Source: CAD feature listing. Evaluate the final solid. Frame: model axes, mm. Coordinates: 2 decimals unless noted, no trailing zeros. Loops run counter-clockwise (first coordinate to the right, second up) from the corner with the lowest first, then second, coordinate; pieces in that order, holes last. Notation, with made-up numbers: (69.25, 59.5) -> (117.25, 59.5) arc R23 ccw to (117.25, 79.5) -> close; hole circle Ø4 at (13.5, 29). An arc over 180 degrees is marked (long way). One line per question, with ' | ' between items. Start each with the question number.
```python
from build123d import *

# Parameters (mm, degrees)
SKETCH1_R           = 38.1
SKETCH1_R_2         = 36.83
BOSS_EXTRUDE1_DEPTH = 254
CUT_EXTRUDE1_DEPTH  = 260.652113413
CIRPATTERN1_COUNT   = 2
CIRPATTERN1_ANGLE   = 90


with BuildPart() as part:
    # Sketch1 → Boss-Extrude1 (new body)
    with BuildSketch(Plane(origin=(0, 0, 0), x_dir=(1, 0, 0), z_dir=(0, 1, 0))):
        with Locations(Location((0, 0, 0), (0, 0, 270))):
            Circle(SKETCH1_R)
        with Locations(Location((0, 0, 0), (0, 0, 270))):
            Circle(SKETCH1_R_2, mode=Mode.SUBTRACT)
    extrude(amount=BOSS_EXTRUDE1_DEPTH)

    # Sketch2 → Cut-Extrude1 (cut, symmetric)
    with BuildSketch(Plane.XY):
        with BuildLine():
            Line((-1.61925, 12.7), (-1.61925, 107.823))
            ThreePointArc((-1.61925, 107.823), (0, 109.44225), (1.61925, 107.823))
            Line((1.61925, 107.823), (1.61925, 12.7))
            ThreePointArc((1.61925, 12.7), (0, 11.08075), (-1.61925, 12.7))
        make_face()
    cut_extrude1 = extrude(amount=CUT_EXTRUDE1_DEPTH, both=True, mode=Mode.SUBTRACT)

    # CirPattern1: Cut-Extrude1 ×2 about axis
    cirpattern1_axis = Axis((0, -12.7, 0), (0, 1, 0))
    for i in range(1, CIRPATTERN1_COUNT):
        add(cut_extrude1.rotate(cirpattern1_axis, i * CIRPATTERN1_ANGLE / (CIRPATTERN1_COUNT - 1)), mode=Mode.SUBTRACT)


solid = part.part
```
(1) Draft query along Z for faces 1 (the cylindrical face through (-23.183, 125.222, -30.235)), 2 (the cylindrical face through (-22.41, 125.222, -29.227)), 3 (the flat face through (31.2, 0, -19.9)). Return one class per face: pulls with the +Z half, pulls with the -Z half, needs draft (parallel to the pull), parting line crosses it, or undercut.
(2) Cut plane A-A, the plane y = 95. Return the cut outline in (x, z).
(3) Cut plane B-B, the plane x = 16. Return the cut outline in (y, z).
(4) Contact query for flat-ended pins moving along their axis: pin 1 Ø1.5 at (y, z) = (83.5, 24) entering from -X; pin 2 Ø12 at (x, y) = (-17.5, 81) entering from +Z; pin 3 Ø12 at (y, z) = (227.5, 27.5) entering from +X. Output: stop coordinate, or through.
(5) Cut plane C-C, the plane z = 33. Return the cut outline in (x, y), and give its area (3 significant figures).
(6) Ray query, L1, parallel to X at y = 141, z = 0; L2, parallel to X at y = 66.5, z = 24. Return the intervals inside material, ascending.
(7) Cut plane D-D, the plane y = 208.5. Return the cut outline in (x, z).
Here are the results:
1) face 1: parting line crosses it | face 2: undercut | face 3: needs draft
2) outline: (-38.07, -1.62) arc R38.1 ccw to (-1.62, -38.07) -> (-1.62, -36.79) arc R36.83 cw to (-36.79, -1.62) -> close; (-38.07, 1.62) -> (-36.79, 1.62) arc R36.83 cw to (-1.62, 36.79) -> (-1.62, 38.07) arc R38.1 ccw to start; (1.62, -38.07) arc R38.1 ccw to (38.07, -1.62) -> (36.79, -1.62) arc R36.83 cw to (1.62, -36.79) -> close; (1.62, 36.79) arc R36.83 cw to (36.79, 1.62) -> (38.07, 1.62) arc R38.1 ccw to (1.62, 38.07) -> close
3) outline: (0, -34.58) -> (254, -34.58) -> (254, -33.17) -> (0, -33.17) -> close; (0, 33.17) -> (254, 33.17) -> (254, 34.58) -> (0, 34.58) -> close
4) pin 1: stops at x = -30.18 | pin 2: stops at z = 36.32 | pin 3: stops at x = 31.45
5) outline: (-19.04, 0) -> (-16.35, 0) -> (-16.35, 254) -> (-19.04, 254) -> close; (16.35, 0) -> (19.04, 0) -> (19.04, 254) -> (16.35, 254) -> close | area: 1,370 mm2
6) L1: x = -38.1 to -36.83, 36.83 to 38.1 | L2: x = -29.59 to -27.94, 27.94 to 29.59
7) outline: circle Ø76.2 at (0, 0); hole circle Ø73.66 at (0, 0)
